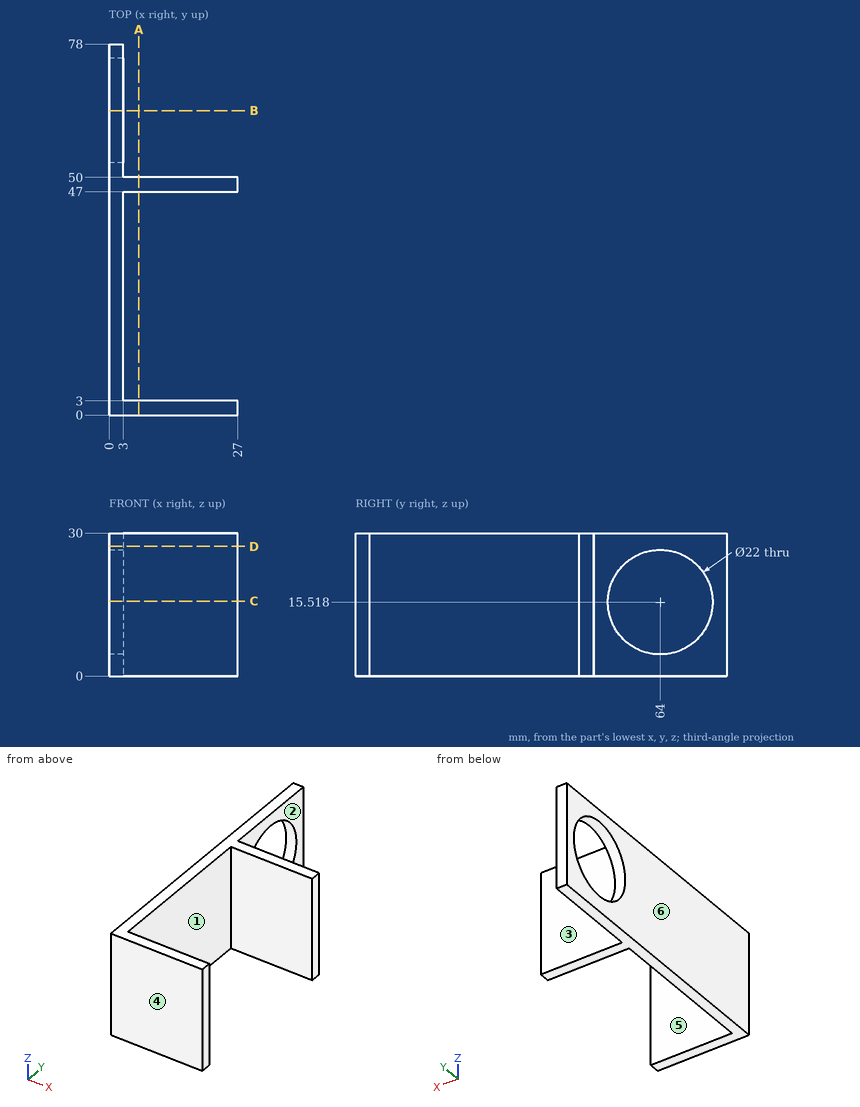
Could you check a few things on this drawing? It's one solid part, dimensions in mm from its lowest x, y, z. A direction names the side the tool comes from. Give positions to 0.01 mm unless a question says otherwise; leave off trailing zeros. Write each loop counter-clockwise with the first axis right and the second up, starting at its lowest first coordinate (ties: lowest second). Pieces come first, ordered by that corner, then holes. Notation, with made-up numbers: (36.25, -20) -> (53.25, -20) arc R28 ccw to (53.25, -2) -> close; hole circle Ø11 at (22, 36). An arc over 180 degrees is marked (long way). Write item = value, one per line.
(1) Thinking about a two-plate mould opening in Y: for the marked faces 1, 2, 3 and 4, which applies, released by +Y, released by -Y, zero draft, split by the parting line, or undercut?
Worked out:
face_1 = undercut
face_2 = zero draft
face_3 = released by +Y
face_4 = released by -Y
(2) Suppose I cut it at C-C on z = 15.75. Write out the boundary of the cut face in (x, y), then the cut area to 3 significant figures.
Worked out:
outline = (0, 0) -> (27, 0) -> (27, 3) -> (3, 3) -> (3, 47) -> (27, 47) -> (27, 50) -> (3, 50) -> (3, 53) -> (0, 53) -> close; (0, 75) -> (3, 75) -> (3, 78) -> (0, 78) -> close
area = 312 mm^2
(3) Suppose I cut it at D-D on z = 27.25. Write out the boundary of the cut face in (x, y), then the cut area to 3 significant figures.
Worked out:
outline = (0, 0) -> (27, 0) -> (27, 3) -> (3, 3) -> (3, 47) -> (27, 47) -> (27, 50) -> (3, 50) -> (3, 78) -> (0, 78) -> close
area = 378 mm^2
(4) I need wall thicknesses on probe 1 along Y at (x, z) = (4.75, 13.5); probe 2 along X at (y, z) = (52.5, 17.75); probe 3 along Y at (x, z) = (2.5, 16.5). Which ranges of each line are inside material? Lowest first, please. Write a range as from..to.
Worked out:
probe_1 = 0..3, 47..50
probe_2 = 0..3
probe_3 = 0..53.04, 74.96..78
(5) Suppose I cut it at B-B on y = 64. Write out the boundary of the cut face in (x, z), then the cut area to 3 significant figures.
Worked out:
outline = (0, 0) -> (3, 0) -> (3, 4.52) -> (0, 4.52) -> close; (0, 26.52) -> (3, 26.52) -> (3, 30) -> (0, 30) -> close
area = 24.0 mm^2
(6) Suppose I cut it at A-A on x = 6.25. Write out the boundary of the cut face in (y, z), then the cut area to 3 significant figures.
Worked out:
outline = (0, 0) -> (3, 0) -> (3, 30) -> (0, 30) -> close; (47, 0) -> (50, 0) -> (50, 30) -> (47, 30) -> close
area = 180 mm^2
(7) I'm going to push flat-ended pins straight in: P1, Ø7, axis at x = 9.5, z = 17.5, coming from the +Y side; P2, Ø8.5, axis at y = 68.5, z = 19, coming from the +X side; P3, Ø1.5, axis at x = 12.5, z = 10, coming from the -Y side; P4, Ø9, axis at y = 26.5, z = 10, coming from the +X side. Where does each tip first touch, or does it pass through?
Worked out:
P1 = 50
P2 = through
P3 = 0
P4 = 3
(8) For the marked faces 5 and 6, which set-ups out of +Z, -Z, +X, -X, +Y, -Y let a thin tool reach every point of the face, with its end or its side?
Worked out:
face_5 = +Z, -Z, +X
face_6 = +Z, -Z, -X, +Y, -Y
